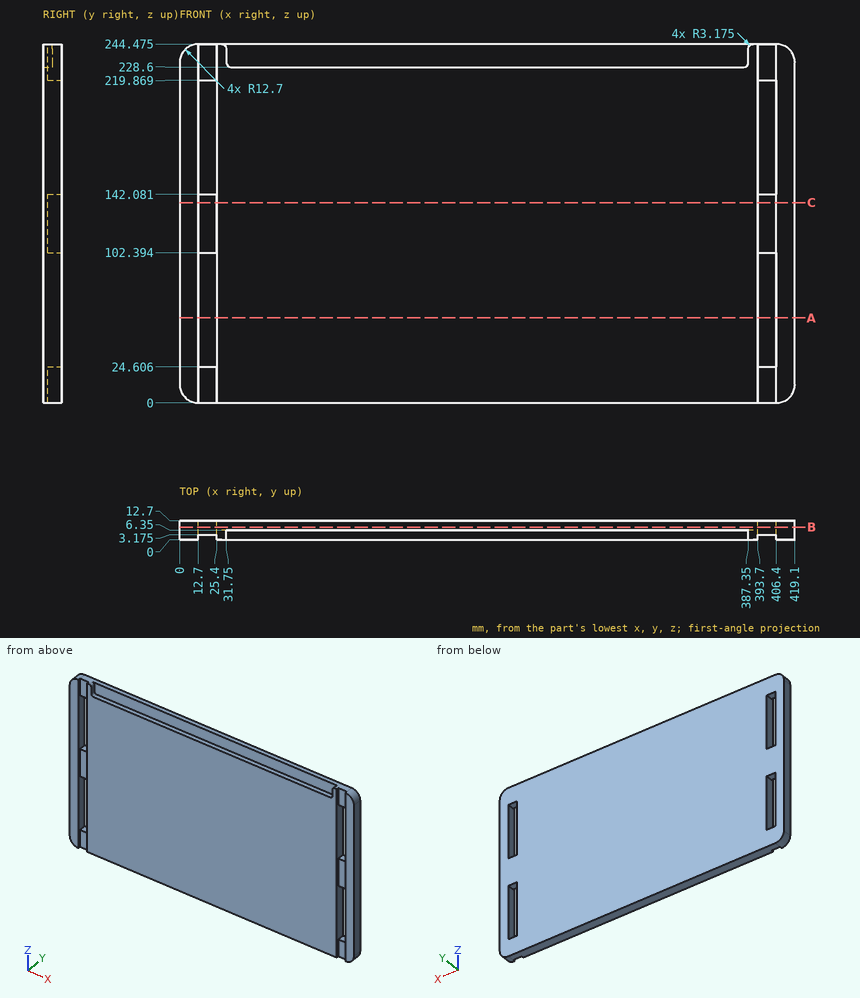
Job drawing, mm, ordinate dimensions from the low corner. One solid piece. Round coordinates to 2 decimals unless told otherwise and drop trailing zeros. Loops run counter-clockwise (first coordinate to the right, second up) from the corner with the lowest first, then second, coordinate; pieces in that order, holes last. Notation, with made-up numbers: (-22.75, 6) -> (29.25, 6) arc R19 cw to (29.25, 40) -> close; hole circle Ø3 at (63, 5). An arc over 180 degrees is marked (long way). One line per item, written item: value. Start each with the question number.
Q1. Cut at C-C on z = 136.5. List the corners of the cut face in (x, y) (1 decimal), plus the area to 3 significant figures.
Q2. Probe line 1 along X through (y, z) = (8.5, 194); line 2 along Z through (x, y) = (55, 2.5); line 3 along Y through (x, z) = (142, 232.5). List the from-to ranges inside material, lowest first.
Q3. Cut at A-A on z = 58. List the corners of the cut face in (x, y), plus the area to 3 significant figures.
Q4. Drop flat-ended pins along their axis: pin 1 Ø4 at (x, z) = (403, 9) entering from -Y (3 decimals); pin 2 Ø7 at (y, z) = (4, 237.5) entering from -X; pin 3 Ø1.9 at (y, z) = (4, 238) entering from +X. Give the stop position or say it passes through.
Q5. Cut at B-B on y = 8.5. List the corners of the cut face in (x, z) (1 decimal), plus the area to 3 significant figures.
Computed:
1. outline: (0, 0) -> (12.7, 0) -> (12.7, 3.2) -> (25.4, 3.2) -> (25.4, 0) -> (393.7, 0) -> (393.7, 3.2) -> (406.4, 3.2) -> (406.4, 0) -> (419.1, 0) -> (419.1, 12.7) -> (0, 12.7) -> close
1. area: 5,240 mm²
2. line 1: 0 to 12.7, 25.4 to 393.7, 406.4 to 419.1
2. line 2: 0 to 228.6
2. line 3: 6.35 to 12.7
3. outline: (0, 0) -> (12.7, 0) -> (12.7, 12.7) -> (0, 12.7) -> close; (25.4, 0) -> (393.7, 0) -> (393.7, 12.7) -> (25.4, 12.7) -> close; (406.4, 0) -> (419.1, 0) -> (419.1, 12.7) -> (406.4, 12.7) -> close
3. area: 5,000 mm²
4. pin 1: y = 3.175
4. pin 2: x = 0.2
4. pin 3: x = 417.95
5. outline: (0, 12.7) arc R12.7 ccw to (12.7, 0) -> (406.4, 0) arc R12.7 ccw to (419.1, 12.7) -> (419.1, 231.8) arc R12.7 ccw to (406.4, 244.5) -> (12.7, 244.5) arc R12.7 ccw to (0, 231.8) -> close; hole (12.7, 24.6) -> (25.4, 24.6) -> (25.4, 102.4) -> (12.7, 102.4) -> close; hole (12.7, 142.1) -> (25.4, 142.1) -> (25.4, 219.9) -> (12.7, 219.9) -> close; hole (393.7, 24.6) -> (406.4, 24.6) -> (406.4, 102.4) -> (393.7, 102.4) -> close; hole (393.7, 142.1) -> (406.4, 142.1) -> (406.4, 219.9) -> (393.7, 219.9) -> close
5. area: 98,400 mm²
